Input: part model. Units: mm. Frame: model coordinates. Round coordinates to 2 decimals unless told otherwise and drop trailing zeros. Order: outer loops, then holes, each group sorted by start corner. A loop starts at its lowest first (then second) coordinate and runs counter-clockwise, first axis right, second up. Notation, with made-up numbers: (33.5, 11) -> (90.5, 11) arc R26 cw to (90.5, 25) -> close; hole circle Ø3 at (-19.5, 55). An arc over 180 degrees is marked (long way). Use a Markdown table: item, result.
from build123d import *


with BuildPart() as part:
    # Croquis1 → Revolución1 (revolve)
    with BuildSketch(Plane(origin=(0, 0, 0), x_dir=(0, 0, -1), z_dir=(1, 0, 0))):
        with BuildLine():
            Line((2.5, -2.4), (2.5, 2.4))
            ThreePointArc((2.5, 2.4), (2.529289322, 2.470710678), (2.6, 2.5))
            Line((2.6, 2.5), (3.5, 2.5))
            Line((3.5, 2.5), (3.5, 2.3))
            Line((3.5, 2.3), (4.5, 2.3))
            Line((4.5, 2.3), (4.5, 2.5))
            Line((4.5, 2.5), (5.4, 2.5))
            ThreePointArc((5.4, 2.5), (5.470710678, 2.470710678), (5.5, 2.4))
            Line((5.5, 2.4), (5.5, -2.4))
            ThreePointArc((5.5, -2.4), (5.470710678, -2.470710678), (5.4, -2.5))
            Line((5.4, -2.5), (4.779574592, -2.5))
            Line((4.779574592, -2.5), (4.779574592, -2.3))
            Line((4.779574592, -2.3), (3.220425408, -2.3))
            Line((3.220425408, -2.3), (3.220425408, -2.5))
            Line((3.220425408, -2.5), (2.6, -2.5))
            ThreePointArc((2.6, -2.5), (2.529289322, -2.470710678), (2.5, -2.4))
        make_face()
    revolve(axis=Axis((0, -2.255244755, 0), (0, 1, 0)))


solid = part.part
1) Line query: L1, parallel to Z at x = 0, y = 2.4; L2, parallel to X at y = -2.4, z = 0. Output: solid intervals per line, ascending. Write a range as [from, to].
Results found:
| item | result |
|---|---|
| L1 | z = [-5.5, -4.5], [-3.5, -2.5], [2.5, 3.5], [4.5, 5.5] |
| L2 | x = [-5.5, -4.78], [-3.22, -2.5], [2.5, 3.22], [4.78, 5.5] |
2) Pull-direction query (X, two-part tool) for faces 1 (the flat face through (-3, 2.5, 0)), 2 (the flat face through (4, 2.3, 0)), 3 (the cylindrical face through (5.37, -0.03, 1.19)); classes: +X half, -X half, draft (parallel to the pull), parting line (faces both ways), or undercut.
Results found:
| item | result |
|---|---|
| face 1 | draft |
| face 2 | undercut |
| face 3 | parting line |
3) Pin query (flat end, axial travel): pin 1 Ø2 at (y, z) = (0.5, -2.5) entering from -X; pin 2 Ø1.5 at (y, z) = (-1, -3.5) entering from +X. Return the tip coordinate at first contact, or that it passes through.
Results found:
| item | result |
|---|---|
| pin 1 | stops at x = -5.29 |
| pin 2 | stops at x = 4.76 |
4) Cut plane C-C on y = 1.8. Return loops of the section in (x, z), and give its area (3 significant figures).
Results found:
| item | result |
|---|---|
| outline | circle Ø11 at (0, 0); hole circle Ø5 at (0, 0) |
| area | 75.4 mm² |
